from build123d import *

# Parameters (mm, degrees)
SKETCH1_R           = 1.5875
BOSS_EXTRUDE1_DEPTH = 0.8128
FILLET1_R           = 0.4064


with BuildPart() as part:
    # Sketch1 → Boss-Extrude1 (new body)
    with BuildSketch(Plane.XY):
        with BuildLine():
            Line((0, -0.8128), (65.4074384, -0.8128))
            Line((65.4074384, -0.8128), (65.4074384, 0))
            Line((65.4074384, 0), (70.1699384, 0))
            Line((70.1699384, 0), (70.1699384, -0.8128))
            Line((70.1699384, -0.8128), (76.5199384, -0.8128))
            Line((76.5199384, -0.8128), (76.5199384, 0))
            Line((76.5199384, 0), (81.2824384, 0))
            Line((81.2824384, 0), (81.2824384, 6.35))
            Line((81.2824384, 6.35), (11.1125, 11.1125))
            ThreePointArc((11.1125, 11.1125), (7.744903955, 12.507403955), (6.35, 15.875))
            ThreePointArc((6.35, 15.875), (3.175, 19.05), (0, 15.875))
            Line((0, 15.875), (0, -0.8128))
        make_face()
        with Locations((3.175, 3.96875)):
            Circle(SKETCH1_R, mode=Mode.SUBTRACT)
        with Locations((3.175, 15.08125)):
            Circle(SKETCH1_R, mode=Mode.SUBTRACT)
    extrude(amount=BOSS_EXTRUDE1_DEPTH)

    # Fillet1
    fillet1_edges = [part.edges().sort_by_distance(p)[0] for p in [
        (81.2824384, 6.35, 0.4064),
        (81.2824384, 0, 0.4064),
        (76.5199384, 0, 0.4064),
        (76.5199384, -0.8128, 0.4064),
        (70.1699384, -0.8128, 0.4064),
        (70.1699384, 0, 0.4064),
        (65.4074384, 0, 0.4064),
        (65.4074384, -0.8128, 0.4064),
        (0, -0.8128, 0.4064),
    ]]
    fillet(fillet1_edges, radius=FILLET1_R - 0.0001)  # a hair under: the kernel refuses the full size


solid = part.part
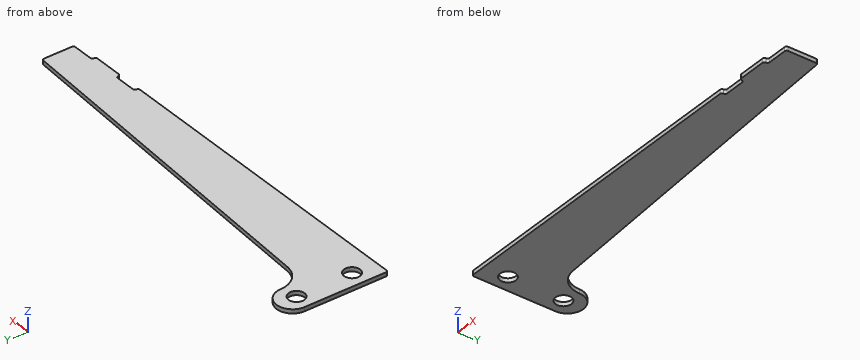
Part model, mm, in its own coordinate system. Round coordinates to 2 decimals unless told otherwise and drop trailing zeros. Order: outer loops, then holes, each group sorted by start corner. A loop starts at its lowest first (then second) coordinate and runs counter-clockwise, first axis right, second up. Notation, with made-up numbers: (-34, 47.5) -> (-16, 47.5) arc R17 ccw to (-16, 53.5) -> close; hole circle Ø1 at (55.25, 78.5). An arc over 180 degrees is marked (long way). Put each result on its own line as item: value.
Q1. Band-saw the part on B-B (x = 54.5). Give the cut face in (y, z).
From the geometry:
outline: (-0.81, 0) -> (8.17, 0) -> (8.17, 0.81) -> (-0.81, 0.81) -> close
Q2. Band-saw the part on C-C (y = 7.5). Give the cut face in (x, z).
From the geometry:
outline: (0, 0) -> (64.34, 0) -> (64.34, 0.81) -> (0, 0.81) -> close
Q3. Wall check: line 1 (X direction, y = 15.25, z = 0.75); line 2 (X direction, y = 6, z = 0.55); line 3 (X direction, y = 13.75, z = 0.4). Give the ranges that are in metal, low to high. Write a range as [from, to].
From the geometry:
line 1: x = [0, 1.6], [4.75, 6.39]
line 2: x = [0, 81.28]
line 3: x = [0, 2.31], [4.04, 6.85]
Q4. Band-saw the part on A-A (z = 0.4). State how many separate pieces and enclosed holes the cut face has, and give its area (3 significant figures).
From the geometry:
separate pieces: 1
enclosed holes: 2
area: 829 mm2
